Input: part model. Units: mm. Frame: model coordinates. A direction names the side the tool comes from. Give positions to 0.01 mm unless a question says otherwise; leave off trailing zeros. Loops run counter-clockwise (first coordinate to the right, second up) from the corner with the lowest first, then second, coordinate; pieces in that order, holes last. Notation, with made-up numbers: (-20.5, -10) - (12.5, -10) arc R19 ccw to (12.5, 9) - close; hole circle Ø7 at (62, 12). An arc over 180 degrees is marked (long way). Answer as a JSON object with one key per item and string values.
from build123d import *

# Parameters (mm, degrees)
F1_DEPTH = 15
F2_DEPTH = 25
F3_DEPTH = 25
F4_R     = 4
F5_DEPTH = 9
F6_R     = 3.2
F7_DEPTH = 13.5
F8_R     = 2
F9_SIZE  = 1


# Not quite as in the source:
# - a feature names something its author has since deleted; it is built from what else it names


with BuildPart() as f1:
    # F0 (on Top) → F1 (new body)
    with BuildSketch(Plane.XY):
        with BuildLine():
            Line((-30, -1.25), (-30, -15))
            Line((-30, -15), (30, -15))
            Line((30, -15), (30, 15))
            Line((30, 15), (-12, 15))
            Line((-12, 15), (-12, 9))
            Line((-12, 9), (-30, 9))
            Line((-30, 9), (-30, 1.25))
            Line((-30, 1.25), (-11.1936553667, 1.25))
            ThreePointArc((-11.1936553667, 1.25), (-5.3253080696, 6), (0.5430392276, 1.25))
            Line((0.5430392276, 1.25), (2.5825958991, 1.25))
            ThreePointArc((2.5825958991, 1.25), (21.5, 0), (2.5825958991, -1.25))
            Line((2.5825958991, -1.25), (0.5430392276, -1.25))
            ThreePointArc((0.5430392276, -1.25), (-5.3253080696, -6), (-11.1936553667, -1.25))
            Line((-11.1936553667, -1.25), (-30, -1.25))
        make_face()
    extrude(amount=F1_DEPTH)

    # F0 (on Top) + F1_face (on face) → F2 (join)
    with BuildSketch(Plane.XY):
        with BuildLine():
            Line((-30, -1.25), (-30, -15))
            Line((-30, -15), (30, -15))
            Line((30, -15), (30, 15))
            Line((30, 15), (-12, 15))
            Line((-12, 15), (-12, 9))
            Line((-12, 9), (-30, 9))
            Line((-30, 9), (-30, 1.25))
            Line((-30, 1.25), (-11.1936553667, 1.25))
            ThreePointArc((-11.1936553667, 1.25), (-5.3253080696, 6), (0.5430392276, 1.25))
            Line((0.5430392276, 1.25), (2.5825958991, 1.25))
            ThreePointArc((2.5825958991, 1.25), (21.5, 0), (2.5825958991, -1.25))
            Line((2.5825958991, -1.25), (0.5430392276, -1.25))
            ThreePointArc((0.5430392276, -1.25), (-5.3253080696, -6), (-11.1936553667, -1.25))
            Line((-11.1936553667, -1.25), (-30, -1.25))
        make_face()
    with BuildSketch(Plane(origin=(0.3427711831, -1.0419373609, 0), x_dir=(1, 0, 0), z_dir=(0, 0, -1))):
        with BuildLine():
            ThreePointArc((2.239824716, 0.2080626391), (21.1572288169, -1.0419373609), (2.239824716, -2.2919373609))
            Line((2.239824716, -2.2919373609), (0.2002680445, -2.2919373609))
            ThreePointArc((0.2002680445, -2.2919373609), (-5.6680792527, -7.0419373609), (-11.5364265498, -2.2919373609))
            Line((-11.5364265498, -2.2919373609), (-30.3427711831, -2.2919373609))
            Line((-30.3427711831, -2.2919373609), (-30.3427711831, -10.0419373609))
            Line((-30.3427711831, -10.0419373609), (-12.3427711831, -10.0419373609))
            Line((-12.3427711831, -10.0419373609), (-12.3427711831, -16.0419373609))
            Line((-12.3427711831, -16.0419373609), (29.6572288169, -16.0419373609))
            Line((29.6572288169, -16.0419373609), (29.6572288169, 13.9580626391))
            Line((29.6572288169, 13.9580626391), (-30.3427711831, 13.9580626391))
            Line((-30.3427711831, 13.9580626391), (-30.3427711831, 0.2080626391))
            Line((-30.3427711831, 0.2080626391), (-11.5364265498, 0.2080626391))
            ThreePointArc((-11.5364265498, 0.2080626391), (-5.6680792527, 4.9580626391), (0.2002680445, 0.2080626391))
            Line((0.2002680445, 0.2080626391), (2.239824716, 0.2080626391))
        make_face()
    extrude(amount=F2_DEPTH, dir=(0, 0, 1))

    # F0 (on Top) → F3 (join)
    with BuildSketch(Plane.XY):
        with BuildLine():
            Line((-30, -1.25), (-30, -15))
            Line((-30, -15), (30, -15))
            Line((30, -15), (30, 15))
            Line((30, 15), (-12, 15))
            Line((-12, 15), (-12, 9))
            Line((-12, 9), (-30, 9))
            Line((-30, 9), (-30, 1.25))
            Line((-30, 1.25), (-11.1936553667, 1.25))
            ThreePointArc((-11.1936553667, 1.25), (-5.3253080696, 6), (0.5430392276, 1.25))
            Line((0.5430392276, 1.25), (2.5825958991, 1.25))
            ThreePointArc((2.5825958991, 1.25), (21.5, 0), (2.5825958991, -1.25))
            Line((2.5825958991, -1.25), (0.5430392276, -1.25))
            ThreePointArc((0.5430392276, -1.25), (-5.3253080696, -6), (-11.1936553667, -1.25))
            Line((-11.1936553667, -1.25), (-30, -1.25))
        make_face()
    extrude(amount=F3_DEPTH)

    # F4 (on face) → F5 (cut)
    with BuildSketch(Plane(origin=(0, 9, 0), x_dir=(-1, 0, 0), z_dir=(0, 1, 0))):
        with Locations((22, 12.5)):
            Circle(F4_R)
    extrude(amount=-F5_DEPTH, mode=Mode.SUBTRACT)

    # F6 (on face) → F7 (cut)
    with BuildSketch(Plane.XZ.offset(15)):
        with Locations((-22, 12.5)):
            Circle(F6_R)
    extrude(amount=-F7_DEPTH, mode=Mode.SUBTRACT)

    # F8
    f8_edges = [f1.edges().sort_by_distance(p)[0] for p in [
        (30, -15, 12.5),
        (30, 15, 12.5),
        (-30, -15, 12.5),
        (-30, 9, 12.5),
    ]]
    fillet(f8_edges, radius=F8_R)

    # F9
    f9_edges = [f1.edges().sort_by_distance(p)[0] for p in [
        (-30, -7.125, 0),
        (-29.414214, -14.414214, 0),
        (-20.596828, -1.25, 0),
        (0, -15, 0),
        (-5.325308, -6, 0),
        (29.414214, -14.414214, 0),
        (1.562818, -1.25, 0),
        (30, 0, 0),
        (21.5, 0, 0),
        (29.414214, 14.414214, 0),
        (1.562818, 1.25, 0),
        (8, 15, 0),
        (-5.325308, 6, 0),
        (-12, 12, 0),
        (-20.596828, 1.25, 0),
        (-20, 9, 0),
        (-30, 4.125, 0),
        (-29.414214, 8.414214, 0),
    ]]
    chamfer(f9_edges, length=F9_SIZE)


solid = f1.part
Item 1: Material intervals for line 1 (Y direction, x = -15, z = 9.5); line 2 (Y direction, x = 12, z = 12); line 3 (X direction, y = -8, z = 11), sorted ascending. Write a range as [from, to].
Geometry check:
{"line 1": "y = [-15, -1.25], [1.25, 9]", "line 2": "y = [-15, -9.5], [9.5, 15]", "line 3": "x = [-30, -24.83], [-19.17, 6.88], [17.12, 30]"}
Item 2: Contact query for flat-ended pins moving along their axis: P1, Ø15, axis at x = -21, z = 9.5, coming from the -Y side; P2, Ø8, axis at x = -19, z = 10.5, coming from the +Y side; P3, Ø5, axis at x = -22, z = 12.5, coming from the -Y side; P4, Ø5, axis at y = 10.5, z = 18.5, coming from the -X side. Output: stop coordinate, or through.
Geometry check:
{"P1": "stops at y = -15", "P2": "stops at y = 9", "P3": "stops at y = -1.5", "P4": "stops at x = -29.73"}
Item 3: Cut plane B-B (x = 12). Return loops of the section in (y, z).
Geometry check:
{"outline": "(-15, 1) - (-14, 0) - (-10.5, 0) - (-9.5, 1) - (-9.5, 25) - (-15, 25) - close; (9.5, 1) - (10.5, 0) - (14, 0) - (15, 1) - (15, 25) - (9.5, 25) - close"}
Item 4: Cut plane D-D (y = 0). Return loops of the section in (x, z), then the cut area to 4 significant figures.
Geometry check:
{"outline": "(21.5, 1) - (22.5, 0) - (29, 0) - (30, 1) - (30, 25) - (21.5, 25) - close", "area": "211.5 mm2"}
Item 5: Access query for faces 1 (the face through (-25.2, -8.3, 12.6)), 2 (the face through (-5.4, 6.2, 0.8)), 3 (the face through (-20, -1.25, 13)), 4 (the face through (-18, 9, 15)), 5 (the face through (0, -15, 13)). Directions: +Z, -Z, +X, -X, +Y, -Y. A direction counts if a zero-diameter tool reaches every point of the face in a straight line with its end or side. Return the directions, or none.
Geometry check:
{"face 1": "-Y", "face 2": "-Z", "face 3": "+Z, -Z, -X", "face 4": "+Z, -Z, -X, +Y", "face 5": "+Z, -Z, +X, -X, -Y"}
Item 6: Cut plane A-A (x = -22). Return loops of the section in (y, z).
Geometry check:
{"outline": "(-15, 1) - (-14, 0) - (-2.25, 0) - (-1.25, 1) - (-1.25, 25) - (-15, 25) - (-15, 15.7) - (-1.5, 15.7) - (-1.5, 9.3) - (-15, 9.3) - close; (1.25, 1) - (2.25, 0) - (8, 0) - (9, 1) - (9, 8.5) - (1.25, 8.5) - close; (1.25, 16.5) - (9, 16.5) - (9, 25) - (1.25, 25) - close"}
Item 7: Mould query, pull axis Y, two halves, no side actions, for faces 6 (the face through (-29.43, -14.4, 13.17)), 7 (the face through (-29.4, 8.43, 13.17)), 8 (the face through (0, -6, 0)), 9 (the face through (-18.6, 1.25, 15.5)). Classes: released by +Y, released by -Y, zero draft, split by the parting line, or undercut.
Geometry check:
{"face 6": "released by -Y", "face 7": "released by +Y", "face 8": "zero draft", "face 9": "undercut"}
Item 8: Cut plane C-C (z = 14.75). Return loops of the section in (x, y).
Geometry check:
{"outline": "(-30, -13) arc R2 ccw to (-28, -15) - (-24.28, -15) - (-24.28, -1.5) - (-19.72, -1.5) - (-19.72, -15) - (28, -15) arc R2 ccw to (30, -13) - (30, 13) arc R2 ccw to (28, 15) - (-12, 15) - (-12, 9) - (-18.69, 9) - (-18.69, 1.25) - (-11.19, 1.25) arc R6 cw to (0.54, 1.25) - (2.58, 1.25) arc R9.5 cw (long way) to (2.58, -1.25) - (0.54, -1.25) arc R6 cw to (-11.19, -1.25) - (-30, -1.25) - close; (-30, 1.25) - (-25.31, 1.25) - (-25.31, 9) - (-28, 9) arc R2 ccw to (-30, 7) - close"}
